from build123d import *

# Parameters (mm, degrees)
F0_W     = 23.5
F0_H     = 10
F1_DEPTH = 60
F2_W     = 21.615356
F2_H     = 11.912346
F3_DEPTH = 8


with BuildPart() as f1:
    # F0 (on Top) → F1 (new body)
    with BuildSketch(Plane.XY):
        Rectangle(F0_W, F0_H)
    extrude(amount=F1_DEPTH)

    # F2 (on face) → F3 (cut)
    with BuildSketch(Plane.XZ.offset(5)):
        with Locations((0, 52.550074)):
            Rectangle(F2_W, F2_H)
        with Locations((0, 37.576918)):
            Rectangle(F2_W, F2_H)
        with Locations((0, 22.839397)):
            Rectangle(F2_W, F2_H)
        with Locations((0, 8.101878)):
            Rectangle(F2_W, F2_H)
    extrude(amount=-F3_DEPTH, mode=Mode.SUBTRACT)


solid = f1.part
Here's how the part is built. I have some questions about the finished solid (model axes, mm). A direction names the side the tool comes from. Round coordinates to 2 decimals unless told otherwise and drop trailing zeros. Order: outer loops, then holes, each group sorted by start corner. A loop starts at its lowest first (then second) coordinate and runs counter-clockwise, first axis right, second up. Notation, with made-up numbers: (25.25, -7.75) -> (75.25, -7.75) arc R12 ccw to (75.25, 12.25) -> close; hole circle Ø5 at (-5, 23.25). An arc over 180 degrees is marked (long way). Use CSV: the item, a comma, the result in double quotes.
1. I need wall thicknesses on line 1 along Z through (x, y) = (1.5, 0); line 2 along X through (y, z) = (-0.75, 13); line 3 along Y through (x, z) = (10.5, 41). Which ranges of each line are inside material? Lowest first, please.
Recorded:
line 1,"z = 0 to 2.15, 14.06 to 16.88, 28.8 to 31.62, 43.53 to 46.59, 58.51 to 60"
line 2,"x = -11.75 to -10.81, 10.81 to 11.75"
line 3,"y = 3 to 5"
2. I want a section at A-A on y = -0.5. List the corners of the cut face in (x, z) for me, and give its area (3 significant figures).
Recorded:
outline,"(-11.75, 0) -> (11.75, 0) -> (11.75, 60) -> (-11.75, 60) -> close; hole (-10.81, 2.15) -> (10.81, 2.15) -> (10.81, 14.06) -> (-10.81, 14.06) -> close; hole (-10.81, 16.88) -> (10.81, 16.88) -> (10.81, 28.8) -> (-10.81, 28.8) -> close; hole (-10.81, 31.62) -> (10.81, 31.62) -> (10.81, 43.53) -> (-10.81, 43.53) -> close; hole (-10.81, 46.59) -> (10.81, 46.59) -> (10.81, 58.51) -> (-10.81, 58.51) -> close"
area,"380 mm2"
3. Thinking about a two-plate mould opening in Z: for faces 3 (the face through (-10.808, -1, 37)), 4 (the face through (0, 0, 0)), 5 (the face through (0, 5, 30)), which applies, pulls with the +Z half, pulls with the -Z half, needs draft (parallel to the pull), parting line crosses it, or undercut?
Recorded:
face 3,"undercut"
face 4,"pulls with the -Z half"
face 5,"needs draft"
4. I'm going to push a flat-ended pin straight in: P1, Ø6, axis at x = -4.5, z = 9, coming from the -Y side. Where does the tip first touch, or does it pass through?
Recorded:
P1,"stops at y = 3"
5. I want a section at C-C on x = -5.5. List the corners of the cut face in (y, z) for me.
Recorded:
outline,"(-5, 0) -> (5, 0) -> (5, 60) -> (-5, 60) -> (-5, 58.51) -> (3, 58.51) -> (3, 46.59) -> (-5, 46.59) -> (-5, 43.53) -> (3, 43.53) -> (3, 31.62) -> (-5, 31.62) -> (-5, 28.8) -> (3, 28.8) -> (3, 16.88) -> (-5, 16.88) -> (-5, 14.06) -> (3, 14.06) -> (3, 2.15) -> (-5, 2.15) -> close"
6. I want a section at B-B on z = 23. List the corners of the cut face in (x, y) for me, and give its area (3 significant figures).
Recorded:
outline,"(-11.75, -5) -> (-10.81, -5) -> (-10.81, 3) -> (10.81, 3) -> (10.81, -5) -> (11.75, -5) -> (11.75, 5) -> (-11.75, 5) -> close"
area,"62.1 mm2"
7. Which directions (+Z, -Z, +X, -X, +Y, -Y) give clear straight access to the entire face, cutting with the end or side of a thin tool? Please do faces 1 (the face through (10.808, -1, 52)), 2 (the face through (11.75, 0, 30)).
Recorded:
face 1,"-Y"
face 2,"+Z, -Z, +X, +Y, -Y"
